Verification items for the finished model (mm, model axes). Face numbers are marked on the shaded views. A direction names the side the tool comes from. Give positions to 0.01 mm unless a question says otherwise; leave off trailing zeros. Loops run counter-clockwise (first coordinate to the right, second up) from the corner with the lowest first, then second, coordinate; pieces in that order, holes last. Notation, with made-up numbers: (39.25, 28.5) - (98.25, 28.5) arc R28 cw to (98.25, 61.5) - close; hole circle Ø7 at (-24.75, 64). An arc over 180 degrees is marked (long way). Use one line per item in the form item = value.
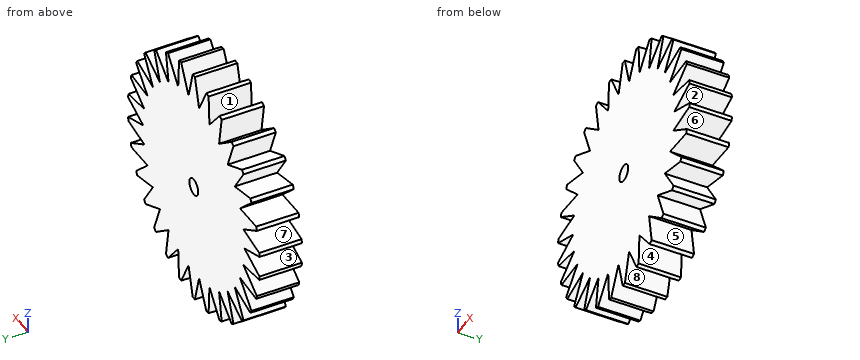
Autodesk Inventor part; units mm, degrees
ref_plane "YZ Plane" through (0, 0, 0) normal (1, 0, 0) x (0, 1, 0)
ref_plane "XZ Plane" through (0, 0, 0) normal (0, 1, 0) x (-1, 0, 0)
ref_plane "XY Plane" through (0, 0, 0) normal (0, 0, 1) x (1, 0, 0)
sketch "Sketch1" plane through (0, 0, 0) normal (0, 1, 0) x (-1, 0, 0)
  circle A0 centre (0, 0) radius 15
  line L0 (14.942, 1.3178) -> (11.506, 0)
  line L1 (11.506, 0) -> (14.942, -1.3178)
  line L2 (14.3415, 4.3956) -> (11.2545, 2.3922)
  line L3 (11.2545, 2.3922) -> (14.8895, 1.8176)
  line L4 (13.1142, 7.2813) -> (10.5112, 4.6799)
  line L5 (10.5112, 4.6799) -> (14.1862, 4.8736)
  line L6 (11.3137, 9.8488) -> (9.3085, 6.763)
  line L7 (9.3085, 6.763) -> (12.8629, 7.7166)
  line L8 (9.0188, 11.9859) -> (7.699, 8.5506)
  line L9 (7.699, 8.5506) -> (10.9775, 10.2223)
  line L10 (6.3297, 13.5991) -> (5.753, 9.9645)
  line L11 (5.753, 9.9645) -> (8.6123, 12.2812)
  line L12 (3.364, 14.6179) -> (3.5555, 10.9428)
  line L13 (3.5555, 10.9428) -> (5.8706, 13.8035)
  line L14 (0.2513, 14.9979) -> (1.2027, 11.4429)
  line L15 (1.2027, 11.4429) -> (2.8725, 14.7224)
  line L16 (-2.8725, 14.7224) -> (-1.2027, 11.4429)
  line L17 (-1.2027, 11.4429) -> (-0.2513, 14.9979)
  line L18 (-5.8706, 13.8035) -> (-3.5555, 10.9428)
  line L19 (-3.5555, 10.9428) -> (-3.364, 14.6179)
  line L20 (-8.6123, 12.2812) -> (-5.753, 9.9645)
  line L21 (-5.753, 9.9645) -> (-6.3297, 13.5991)
  line L22 (-10.9775, 10.2223) -> (-7.699, 8.5506)
  line L23 (-7.699, 8.5506) -> (-9.0188, 11.9859)
  line L24 (-12.8629, 7.7166) -> (-9.3085, 6.763)
  line L25 (-9.3085, 6.763) -> (-11.3137, 9.8488)
  line L26 (-14.1862, 4.8736) -> (-10.5112, 4.6799)
  line L27 (-10.5112, 4.6799) -> (-13.1142, 7.2813)
  line L28 (-14.8895, 1.8176) -> (-11.2545, 2.3922)
  line L29 (-11.2545, 2.3922) -> (-14.3415, 4.3956)
  line L30 (-14.942, -1.3178) -> (-11.506, 0)
  line L31 (-11.506, 0) -> (-14.942, 1.3178)
  line L32 (-14.3415, -4.3956) -> (-11.2545, -2.3922)
  line L33 (-11.2545, -2.3922) -> (-14.8895, -1.8176)
  line L34 (-13.1142, -7.2813) -> (-10.5112, -4.6799)
  line L35 (-10.5112, -4.6799) -> (-14.1862, -4.8736)
  line L36 (-11.3137, -9.8488) -> (-9.3085, -6.763)
  line L37 (-9.3085, -6.763) -> (-12.8629, -7.7166)
  line L38 (-9.0188, -11.9859) -> (-7.699, -8.5506)
  line L39 (-7.699, -8.5506) -> (-10.9775, -10.2223)
  line L40 (-6.3297, -13.5991) -> (-5.753, -9.9645)
  line L41 (-5.753, -9.9645) -> (-8.6123, -12.2812)
  line L42 (-3.364, -14.6179) -> (-3.5555, -10.9428)
  line L43 (-3.5555, -10.9428) -> (-5.8706, -13.8035)
  line L44 (-0.2513, -14.9979) -> (-1.2027, -11.4429)
  line L45 (-1.2027, -11.4429) -> (-2.8725, -14.7224)
  line L46 (2.8725, -14.7224) -> (1.2027, -11.4429)
  line L47 (1.2027, -11.4429) -> (0.2513, -14.9979)
  line L48 (5.8706, -13.8035) -> (3.5555, -10.9428)
  line L49 (3.5555, -10.9428) -> (3.364, -14.6179)
  line L50 (8.6123, -12.2812) -> (5.753, -9.9645)
  line L51 (5.753, -9.9645) -> (6.3297, -13.5991)
  line L52 (10.9775, -10.2223) -> (7.699, -8.5506)
  line L53 (7.699, -8.5506) -> (9.0188, -11.9859)
  line L54 (12.8629, -7.7166) -> (9.3085, -6.763)
  line L55 (9.3085, -6.763) -> (11.3137, -9.8488)
  line L56 (14.1862, -4.8736) -> (10.5112, -4.6799)
  line L57 (10.5112, -4.6799) -> (13.1142, -7.2813)
  line L58 (14.8895, -1.8176) -> (11.2545, -2.3922)
  line L59 (11.2545, -2.3922) -> (14.3415, -4.3956)
  dimension "d0" = 30
  dimension "d3" = 360
extrude "Extrusion1" add sketch "Sketch1" along normal blind 5 contours L0 L1 A0 L58 L59 L56 L57 L54 L55 L52 L53 L50 L51 L48 L49 L46 L47 L44 L45 L42 L43 L40 L41 L38 L39 L36 L37 L34 L35 L32 L33 L30 L31 L28 L29 L26 L27 L24 L25 L22 L23 L20 L21 L18 L19 L16 L17 L14 L15 L12 L13 L10 L11 L8 L9 L6 L7 L4 L5 L2 L3
sketch "Sketch4" plane through (0, 0, 0) normal (0, -1, 0) x (1, 0, 0)
  circle A0 centre (0, 0) radius 1
  dimension "d17" = 2
extrude "Extrusion4" cut sketch "Sketch4" against normal blind 10
properties part number "30ToothGear"
1. Draft check along X on the marked faces 6, 7 and 8. Enter one of: released by +X, released by -X, zero draft, split by the parting line, or undercut.
Result set:
face_6 = released by +X
face_7 = released by -X
face_8 = undercut
2. Section check A-A, the plane z = 9. Record the cut outline in (x, y), then the cut area to 3 significant figures.
Result set:
outline = (-10.76, 0) - (-8.58, 0) - (-8.58, 5) - (-10.76, 5) - close; (-7.87, 0) - (7.87, 0) - (7.87, 5) - (-7.87, 5) - close; (8.58, 0) - (10.76, 0) - (10.76, 5) - (8.58, 5) - close
area = 101 mm²
3. Scan lines: probe 1 along Z at (x, y) = (-12, 3.8); probe 2 along Z at (x, y) = (0, 3.6); probe 3 along X at (y, z) = (4.1, -12.5). Record each from-to range of solid material in increasing order.
Result set:
probe_1 = -7.49 to -6.17, -4.76 to -2.88, -2.27 to -0.19, 0.19 to 2.27, 2.88 to 4.76, 6.17 to 7.49
probe_2 = -15 to -1, 1 to 15
probe_3 = -6.16 to -4.82, -3.47 to -1.74, -0.92 to 0.92, 1.74 to 3.47, 4.82 to 6.16
4. Depth check by flat-ended pin: pin 1 Ø3 at (y, z) = (1, 6.5) entering from +X; pin 2 Ø1.5 at (y, z) = (1, -8) entering from -X. Enter the tip coordinate at first touch or a pass-through.
Result set:
pin_1 = 13.11
pin_2 = -13.11
5. Tool access check on the marked faces 1, 2, 3, 4 and 5. Record the directions out of +Z, -Z, +X, -X, +Y, -Y that give a thin tool (end or side, any length) a straight path to the whole face; none if there is none.
Result set:
face_1 = +Z, +Y, -Y
face_2 = +X, +Y, -Y
face_3 = -X, +Y, -Y
face_4 = -Z, +Y, -Y
face_5 = +Y, -Y
